Autodesk Inventor part; units mm, degrees
ref_plane "YZ Plane" through (0, 0, 0) normal (1, 0, 0) x (0, 1, 0)
ref_plane "XZ Plane" through (0, 0, 0) normal (0, 1, 0) x (-1, 0, 0)
ref_plane "XY Plane" through (0, 0, 0) normal (0, 0, 1) x (1, 0, 0)
sketch "Sketch1" plane through (0, 0, 0) normal (0, 0, 1) x (1, 0, 0)
  line L0 (-21.05, -11.5) -> (21.05, -11.5)
  line L1 (21.05, -11.5) -> (21.05, 11.5)
  line L2 (21.05, 11.5) -> (-21.05, 11.5)
  line L3 (-21.05, 11.5) -> (-21.05, -11.5)
  line L4 (-21.05, -11.5) -> (21.05, 11.5) construction
  line L5 (21.05, -11.5) -> (-21.05, 11.5) construction
  point P0 (0, 0)
  dimension "d0" = 42.1
  dimension "d1" = 23
extrude "Plate1" add sketch "Sketch1" along normal blind 1.5
sketch "Sketch2" plane through (0, 0, 1.5) normal (0, 0, 1) x (1, 0, 0)
  circle A0 centre (17.55, 7.095) radius 0.7835
  circle A1 centre (17.55, -7.955) radius 0.7835
  circle A2 centre (2.45, 7.095) radius 0.7835
  circle A3 centre (2.45, -7.955) radius 0.7835
  circle A4 centre (-17.55, 7.095) radius 0.7835
  circle A5 centre (-17.55, -7.955) radius 0.7835
  point P0 (0, 0)
hole "Hole1" at (17.55, -7.955, 1.5) at (2.45, -7.955, 1.5) at (-17.55, -7.955, 1.5) at (-17.55, 7.095, 1.5) at (2.45, 7.095, 1.5) at (17.55, 7.095, 1.5) direction (0, 0, -1) diameter 2.1 end through all
sketch "Sketch3" plane through (0, 0, 1.5) normal (0, 0, 1) x (1, 0, 0)
  circle A0 centre (-10.05, -0.43) radius 6.4
  circle A1 centre (-10.05, -0.43) radius 6.6
  point P0 (0, 0)
  dimension "d10" = 0.2
extrude "Extrusion1" cut sketch "Sketch3" against normal through all contours A0 | A1
sketch "Sketch4" plane through (-21.05, 10, 0) normal (0, 1, 0) x (-1, 0, 0)
  line L0 (-42.1, 0) -> (0, 0)
  line L1 (0, 0) -> (0, 25)
  line L2 (0, 25) -> (-42.1, 25)
  line L3 (-42.1, 25) -> (-42.1, 0)
edge flange "Flange1" height 25 angle 90 thickness 1.5 bend radius 0.31 thickness toward (0, 1, 0) relief tear relief width 1.5 relief depth 0.75 edges at (0, 11.5, 1.5) wall of the first edge with corners at (21.05, 10, 0) (-21.05, 10, 0) (-21.05, 10, 25) (21.05, 10, 25)
bend "Bend1"
corner "Corner1"
sketch "Sketch5" plane through (-21.05, 10, 25) normal (0, -1, 0) x (1, 0, 0)
  circle A0 centre (21.05, -45.25) radius 40
  circle A1 centre (21.05, -45.25) radius 53
  point P0 (21.05, -25)
  dimension "d23" = 13
extrude "Cut1" cut sketch "Sketch5" against normal blind 1.5
fillet "Corner Round1" radius 1 2 edges at (21.05, -11.5, 0.75) (-21.05, -11.5, 0.75)
sketch "Sketch6" plane through (-21.05, 10, 1.81) normal (0, -1, 0) x (1, 0, 0)
  line L0 (0, 0) -> (42.1, 0)
  arc A0 (42.1, 11.9532) -> (0, 11.9532) centre (21.05, -22.06) ccw
  line L1 (21.05, 0) -> (21.05, 17.94) construction
  point P0 (21.05, -1.81)
  point P1 (3.05, 3)
  point P2 (3.05, 10)
  point P3 (21.05, 13)
  point P4 (21.05, 3)
  point P5 (39.05, 3)
  point P6 (39.05, 10)
  dimension "d27" = 10
  dimension "d28" = 3
  dimension "d29" = 18
  dimension "d30" = 7
hole "Hole2" at (-18, 10, 4.81) at (-18, 10, 11.81) at (0, 10, 14.81) at (0, 10, 4.81) at (18, 10, 4.81) at (18, 10, 11.81) direction (0, 1, 0) diameter 2.1 end through all
equation "\"d8\" = Thickness"
equation "\"d24\" = Thickness"
equation "\"d2\" = Thickness"
equation "\"d13\" = BendReliefWidth"
equation "\"d14\" = BendReliefDepth"
equation "\"d15\" = MinimumRemnant"
equation "\"d16\" = TransitionRadius"
equation "\"d19\" = BendRadius"
equation "\"d20\" = CornerReliefSize"
equation "\"d21\" = GapSize"
equation "\"d22\" = JacobiRadiusSize"
equation "\"BendReliefWidth\" = Thickness"
equation "\"BendReliefDepth\" = 0.5 * Thickness"
equation "\"CornerReliefSize\" = 4 * Thickness"
equation "\"MinimumRemnant\" = 2 * Thickness"
equation "\"TransitionRadius\" = BendRadius"
equation "\"JacobiRadiusSize\" = BendRadius"
equation "\"GapSize\" = Thickness"
properties part number "axis_2_bottom_L_frame(bottom)" material "Aluminum 6061-AHC"
The listing builds one solid part. Answer for the finished solid, in the listing's coordinates (mm). A direction names the side the tool comes from. Give positions to 0.01 mm unless a question says otherwise; leave off trailing zeros. Loops run counter-clockwise (first coordinate to the right, second up) from the corner with the lowest first, then second, coordinate; pieces in that order, holes last. Notation, with made-up numbers: M 68,1 L 125,1 A15 ccw 125,5 Z; hole C -32,38.25 d5. An arc over 180 degrees is marked long. Answer as CSV lines item,"result".
Item 1: Which of the six approach directions +Z, -Z, +X, -X, +Y, -Y give full straight-line access (tool end or side, diameter ignored) to faces 1 (the cylindrical face through (-0.05, 10.76, 5.86)), 2 (the flat face through (0, 10, 11))?
Values follow:
face 1,"+Y, -Y"
face 2,"+Z, +X, -X, -Y"
Item 2: The part is cut by section C-C (y = -8.5). Give the vertices of the cut face in (x, z), and give its area (3 significant figures).
Values follow:
outline,"M -21.05,0 L -18.45,0 L -18.45,1.5 L -21.05,1.5 Z; M -16.65,0 L 1.55,0 L 1.55,1.5 L -16.65,1.5 Z; M 3.35,0 L 16.65,0 L 16.65,1.5 L 3.35,1.5 Z; M 18.45,0 L 21.05,0 L 21.05,1.5 L 18.45,1.5 Z"
area,"55.1 mm^2"
Item 3: The mould has two halves that part along Y. Classify faces 3 (the flat face through (0, 11.5, 11)), 4 (the cylindrical face through (-16.525, 7.323, 0.74)), 5 (the cylindrical face through (-17.148, -8.925, 0.74)), 6 (the cylindrical face through (19.025, 10.76, 5.038)): released by +Y, released by -Y, zero draft, split by the parting line, or undercut.
Values follow:
face 3,"released by +Y"
face 4,"undercut"
face 5,"undercut"
face 6,"zero draft"
Item 4: The part is cut by section D-D (x = 0). Give the vertices of the cut face in (y, z).
Values follow:
outline,"M -11.5,0 L 9.69,0 A1.81 ccw 11.5,1.81 L 11.5,3.76 L 10,3.76 L 10,1.81 A0.31 cw 9.69,1.5 L -11.5,1.5 Z; M 10,5.86 L 11.5,5.86 L 11.5,13.76 L 10,13.76 Z; M 10,15.86 L 11.5,15.86 L 11.5,19.75 L 10,19.75 Z"
Item 5: Straight lines are drawn through the part: line 1 along X through (y, z) = (10.5, 11.81); line 2 along Z through (x, y) = (18, 11.05); line 3 along Z through (x, y) = (18, 10.9). For each, find the intervals that lie inside material, in ascending order. Write a range as [from, to].
Values follow:
line 1,"x = [-21.05, -19.05], [-16.95, 16.95], [19.05, 21.05]"
line 2,"z = [0.62, 3.76], [5.86, 10.76], [12.86, 15.47]"
line 3,"z = [0.46, 3.76], [5.86, 10.76], [12.86, 15.47]"
Item 6: Given pin 1 Ø3.5 at (x, z) = (-18, 11.81) entering from -Y; pin 2 Ø3.5 at (x, z) = (-18, 4.81) entering from +Y; pin 3 Ø1.7 at (x, y) = (17.55, -7.955) entering from -Z; pin 4 Ø1.5 at (x, y) = (2.5, 2) entering from +Z, each flat-ended and moving along its own axis, determine where each tip first touches the part or whether it passes through.
Values follow:
pin 1,"stops at y = 10"
pin 2,"stops at y = 11.5"
pin 3,"passes through"
pin 4,"stops at z = 1.5"
Item 7: The part is cut by section B-B (z = 4.81). Give the vertices of the cut face in (x, y), and give its area (3 significant figures).
Values follow:
outline,"M -21.05,10 L -19.05,10 L -19.05,11.5 L -21.05,11.5 Z; M -16.95,10 L -1.05,10 L -1.05,11.5 L -16.95,11.5 Z; M 1.05,10 L 16.95,10 L 16.95,11.5 L 1.05,11.5 Z; M 19.05,10 L 21.05,10 L 21.05,11.5 L 19.05,11.5 Z"
area,"53.7 mm^2"
Item 8: The part is cut by section A-A (z = 11.81). Give the vertices of the cut face in (x, y), and give its area (4 significant figures).
Values follow:
outline,"M -21.05,10 L -19.05,10 L -19.05,11.5 L -21.05,11.5 Z; M -16.95,10 L 16.95,10 L 16.95,11.5 L -16.95,11.5 Z; M 19.05,10 L 21.05,10 L 21.05,11.5 L 19.05,11.5 Z"
area,"56.85 mm^2"
